Autodesk Inventor part; units mm, degrees
ref_plane "YZ Plane" through (0, 0, 0) normal (1, 0, 0) x (0, 1, 0)
ref_plane "XZ Plane" through (0, 0, 0) normal (0, 1, 0) x (-1, 0, 0)
ref_plane "XY Plane" through (0, 0, 0) normal (0, 0, 1) x (1, 0, 0)
sketch "Sketch1" plane through (0, 0, 0) normal (1, 0, 0) x (0, 1, 0)
  circle A0 centre (0, 0) radius 1.5
  line L0 (0, 0) -> (-35.6, 0)
  circle A1 centre (-35.6, 0) radius 1.5
  line L1 (0, 0) -> (0, -51.5)
  circle A2 centre (0, -51.5) radius 1.5
  circle A3 centre (-35.6, -51.5) radius 1.5
  line L2 (0, 0) -> (-35.6, 0)
  line L3 (-35.6, 0) -> (-35.6, -51.5)
  line L4 (-35.6, -51.5) -> (0, -51.5)
  line L5 (0, -51.5) -> (0, 0)
  line L6 (-17.8, 0) -> (-17.8, -51.5)
  line L7 (-17.8, -25.75) -> (-17.8, 0)
  line L8 (-17.8, -12.875) -> (-17.8, -51.5)
  line L9 (-17.8, -25.75) -> (-17.8, -51.5)
  line L10 (-17.8, -38.625) -> (-17.8, -12.875)
  circle A4 centre (-17.8, -12.875) radius 2.25
  circle A5 centre (-17.8, -38.625) radius 2.25
  line L11 (-15.9797, -9.3512) -> (-0.86, 1.229)
  line L12 (-19.6203, -9.3512) -> (-34.74, 1.229)
  line L13 (-15.55, -15.4984) -> (-15.55, -36.0016)
  line L14 (-20.05, -36.0016) -> (-20.05, -15.4984)
  line L15 (-19.6203, -42.1488) -> (-34.74, -52.729)
  line L16 (-21.2808, -38.5117) -> (-36.5185, -50.3141)
  line L17 (-21.2808, -12.9883) -> (-36.5185, -1.1859)
  line L18 (-14.3192, -12.9883) -> (0.9185, -1.1859)
  line L19 (-14.3192, -38.5117) -> (0.9185, -50.3141)
  line L20 (-15.9797, -42.1488) -> (-0.86, -52.729)
  arc A6 (-14.3192, -12.9883) -> (-15.55, -15.4984) centre (-12.375, -15.4984) ccw
  arc A7 (-15.55, -36.0016) -> (-14.3192, -38.5117) centre (-12.375, -36.0016) ccw
  arc A8 (-21.2808, -38.5117) -> (-20.05, -36.0016) centre (-23.225, -36.0016) ccw
  arc A9 (-20.05, -15.4984) -> (-21.2808, -12.9883) centre (-23.225, -15.4984) ccw
  arc A10 (-19.6203, -9.3512) -> (-15.9797, -9.3512) centre (-17.8, -6.7499) ccw
  arc A11 (-15.9797, -42.1488) -> (-19.6203, -42.1488) centre (-17.8, -44.7501) ccw
  line L21 (1.6962, -2.1899) -> (-13.5415, -13.9923)
  arc A12 (-13.5415, -13.9923) -> (-14.28, -15.4984) centre (-12.375, -15.4984) ccw
  line L22 (-14.28, -15.4984) -> (-14.28, -36.0016)
  arc A13 (-14.28, -36.0016) -> (-13.5415, -37.5077) centre (-12.375, -36.0016) ccw
  line L23 (-13.5415, -37.5077) -> (1.6962, -49.3101)
  line L24 (-37.2962, -2.1899) -> (-22.0585, -13.9923)
  arc A14 (-21.32, -15.4984) -> (-22.0585, -13.9923) centre (-23.225, -15.4984) ccw
  line L25 (-21.32, -15.4984) -> (-21.32, -36.0016)
  arc A15 (-22.0585, -37.5077) -> (-21.32, -36.0016) centre (-23.225, -36.0016) ccw
  line L26 (-22.0585, -37.5077) -> (-37.2962, -49.3101)
  line L27 (-1.5881, 2.2695) -> (-16.7078, -8.3107)
  arc A16 (-18.8922, -8.3107) -> (-16.7078, -8.3107) centre (-17.8, -6.7499) ccw
  line L28 (-18.8922, -8.3107) -> (-34.0119, 2.2695)
  circle A17 centre (0, 0) radius 2.77
  circle A18 centre (-17.8, -12.875) radius 3.52
  circle A19 centre (-17.8, -38.625) radius 3.52
  circle A20 centre (-35.6, 0) radius 2.77
  circle A21 centre (-35.6, -51.5) radius 2.77
  circle A22 centre (0, -51.5) radius 2.77
  line L29 (-1.5881, -53.7695) -> (-16.7078, -43.1893)
  arc A23 (-16.7078, -43.1893) -> (-18.8922, -43.1893) centre (-17.8, -44.7501) ccw
  line L30 (-18.8922, -43.1893) -> (-34.0119, -53.7695)
  point P0 (-17.8, -10.625)
  point P1 (-15.55, -12.875)
  point P2 (-15.55, -38.625)
  point P3 (-20.05, -38.625)
  point P4 (-20.05, -12.875)
  point P5 (-17.8, -40.875)
  point P6 (-18.8754, -36.6486)
  point P7 (-18.8754, -14.8514)
  point P8 (-16.7246, -14.8514)
  point P9 (-16.7246, -36.6486)
  point P10 (-34.0119, 2.2695)
  point P11 (1.6962, -49.3101)
  dimension "d0" = 3
  dimension "d1" = 35.6
  dimension "d2" = 51.5
  dimension "d3" = 4.5
  dimension "d4" = 3.175
  dimension "d5" = 1.27
  dimension "d6" = 1.27
  dimension "d7" = 1.27
  dimension "d8" = 1.27
  dimension "d9" = 1.27
  dimension "d10" = 1.27
  dimension "d11" = 1.27
  dimension "d12" = 1.27
  dimension "d13" = 1.27
  dimension "d14" = 1.27
extrude "Extrusion1" add sketch "Sketch1" along normal blind 2.54 contours A0 L11 L0 A17 L1 L18 | A0 L0 L11 | L18 L1 A0 | A0 L1 L18 A17 L11 L0 | L11 A17 L0 | L1 A17 L18 | A17 L11 A10 A18 L6 A16 L27 L0 | L0 L27 A17 | A17 L18 A18 A10 L11 | A17 L21 L1 | L1 L21 A12 L22 A13 L23 A22 L19 A19 L13 A18 L18 A17 | A18 L13 A6 L18 | L18 A6 L13 A18 L6 A4 A10 | A10 L6 A18 | L23 A22 L1 | L13 A19 L6 A18 | L28 A16 L6 A18 A10 L12 A20 L0 | L0 A20 L28 | A10 A18 L6 | L6 A4 A18 L14 A9 L17 A10 | A22 L4 L20 A2 L19 L1 | L1 L19 A22 | A19 L19 A7 L13 | L13 A7 L19 A19 A11 L6 A5 | L6 A19 L14 A18 | A20 L12 L0 | L0 L12 A1 L17 L3 A20 | A18 L17 A20 L12 A10 | L19 A2 L1 | L1 A2 L4 L20 A22 L19 | A22 L20 A11 A19 L19 | L6 A5 A11 A19 L16 A8 L14 | A18 L17 A9 L14 | L14 A19 L16 A21 L3 L26 A15 L25 A14 L24 A20 L17 A18 | L12 A20 L17 L3 A1 L0 | L0 A1 L12 | A20 L3 L24 | A22 L4 L29 A23 L6 A19 A11 L20 | L20 L4 A22 | L29 L4 A22 | L14 A8 L16 A19 | A20 L3 L17 | A2 L20 L4 | A19 L6 A11 | A19 A11 L15 A21 L16 | L3 L17 A1 | L3 A21 L26 | L6 A19 A11 | L6 A23 L30 L4 A21 L15 A11 A19 | A21 L15 L4 A3 L3 L16 | L16 L3 A21 | L3 L16 A3 L15 L4 A21 | L30 A21 L4 | L3 A3 L16 | A21 L4 L15 | L15 A3 L4
sketch "Sketch2" plane through (2.54, 0, 0) normal (1, 0, 0) x (0, 0, -1)
  circle A0 centre (0, 0) radius 1.5
  circle A1 centre (0, 0) radius 1.5
  circle A2 centre (12.875, -17.8) radius 2.25
  circle A3 centre (12.875, -17.8) radius 2.25
  circle A4 centre (38.625, -17.8) radius 2.25
  circle A5 centre (38.625, -17.8) radius 2.25
  circle A6 centre (51.5, 0) radius 1.5
  circle A7 centre (51.5, 0) radius 1.5
  circle A8 centre (51.5, -35.6) radius 1.5
  circle A9 centre (51.5, -35.6) radius 1.5
  circle A10 centre (0, -35.6) radius 1.5
  circle A11 centre (0, -35.6) radius 1.5
  line L0 (13.9923, -13.5415) -> (2.1899, 1.6962)
  arc A12 (2.1899, 1.6962) -> (-2.2695, -1.5881) centre (0, 0) ccw
  arc A13 (2.1899, 1.6962) -> (-2.2695, -1.5881) centre (0, 0) ccw
  arc A14 (53.7695, -1.5881) -> (49.3101, 1.6962) centre (51.5, 0) ccw
  arc A15 (53.7695, -1.5881) -> (49.3101, 1.6962) centre (51.5, 0) ccw
  arc A16 (49.3101, -37.2962) -> (53.7695, -34.0119) centre (51.5, -35.6) ccw
  arc A17 (49.3101, -37.2962) -> (53.7695, -34.0119) centre (51.5, -35.6) ccw
  arc A18 (-2.2695, -34.0119) -> (2.1899, -37.2962) centre (0, -35.6) ccw
  arc A19 (-2.2695, -34.0119) -> (2.1899, -37.2962) centre (0, -35.6) ccw
  arc A20 (15.4984, -21.32) -> (13.9923, -22.0585) centre (15.4984, -23.225) ccw
  arc A21 (15.4984, -21.32) -> (13.9923, -22.0585) centre (15.4984, -23.225) ccw
  arc A22 (8.3107, -18.8922) -> (8.3107, -16.7078) centre (6.7499, -17.8) ccw
  arc A23 (8.3107, -18.8922) -> (8.3107, -16.7078) centre (6.7499, -17.8) ccw
  arc A24 (13.9923, -13.5415) -> (15.4984, -14.28) centre (15.4984, -12.375) ccw
  arc A25 (13.9923, -13.5415) -> (15.4984, -14.28) centre (15.4984, -12.375) ccw
  arc A26 (36.0016, -14.28) -> (37.5077, -13.5415) centre (36.0016, -12.375) ccw
  arc A27 (36.0016, -14.28) -> (37.5077, -13.5415) centre (36.0016, -12.375) ccw
  arc A28 (37.5077, -22.0585) -> (36.0016, -21.32) centre (36.0016, -23.225) ccw
  arc A29 (37.5077, -22.0585) -> (36.0016, -21.32) centre (36.0016, -23.225) ccw
  arc A30 (43.1893, -16.7078) -> (43.1893, -18.8922) centre (44.7501, -17.8) ccw
  arc A31 (43.1893, -16.7078) -> (43.1893, -18.8922) centre (44.7501, -17.8) ccw
  line L1 (2.1899, 1.6962) -> (13.9923, -13.5415)
  line L2 (-2.2695, -1.5881) -> (8.3107, -16.7078)
  line L3 (8.3107, -16.7078) -> (-2.2695, -1.5881)
  line L4 (8.3107, -18.8922) -> (-2.2695, -34.0119)
  line L5 (8.3107, -18.8922) -> (-2.2695, -34.0119)
  line L6 (2.1899, -37.2962) -> (13.9923, -22.0585)
  line L7 (15.4984, -21.32) -> (36.0016, -21.32)
  line L8 (36.0016, -14.28) -> (15.4984, -14.28)
  line L9 (36.0016, -14.28) -> (15.4984, -14.28)
  line L10 (49.3101, 1.6962) -> (37.5077, -13.5415)
  line L11 (49.3101, 1.6962) -> (37.5077, -13.5415)
  line L12 (43.1893, -16.7078) -> (53.7695, -1.5881)
  line L13 (53.7695, -34.0119) -> (43.1893, -18.8922)
  line L14 (43.1893, -18.8922) -> (53.7695, -34.0119)
  line L15 (37.5077, -22.0585) -> (49.3101, -37.2962)
  arc A32 (-4.3506, -32.5556) -> (4.198, -38.8516) centre (0, -35.6) ccw
  line L16 (-4.3506, -32.5556) -> (5.9748, -17.8)
  line L17 (5.9748, -17.8) -> (-4.3506, -3.0444)
  arc A33 (4.198, 3.2516) -> (-4.3506, -3.0444) centre (0, 0) ccw
  line L18 (4.198, 3.2516) -> (15.8097, -11.74)
  line L19 (15.8097, -11.74) -> (35.6903, -11.74)
  line L20 (35.6903, -11.74) -> (47.302, 3.2516)
  arc A34 (55.8506, -3.0444) -> (47.302, 3.2516) centre (51.5, 0) ccw
  line L21 (47.302, -38.8516) -> (35.6903, -23.86)
  line L22 (35.6903, -23.86) -> (15.8097, -23.86)
  line L23 (15.8097, -23.86) -> (4.198, -38.8516)
  arc A35 (-4.3506, -32.5556) -> (4.198, -38.8516) centre (0, -35.6) ccw
  line L24 (35.4996, -11.9862) -> (47.302, 3.2516)
  arc A36 (55.8506, -3.0444) -> (47.302, 3.2516) centre (51.5, 0) ccw
  line L25 (55.8506, -3.0444) -> (45.5252, -17.8)
  line L26 (45.5252, -17.8) -> (55.8506, -32.5556)
  circle A37 centre (51.5, -35.6) radius 5.31
  point P0 (55.8506, -3.0444)
  point P1 (4.198, -38.8516)
  dimension "d17" = 2.54
  dimension "d18" = 2.54
  dimension "d19" = 2.54
extrude "Extrusion2" add sketch "Sketch2" against normal up to surface (2.54 mm away)
fillet "Fillet1" radius 12.7 6 edges at (1.27, -17.8, -5.9748) (1.27, -23.86, -15.8097) (1.27, -23.86, -35.6903) (1.27, -17.8, -45.5252) (1.27, -11.74, -35.6903) (1.27, -11.74, -15.8097)
properties part number "pump mount_3DPrint"
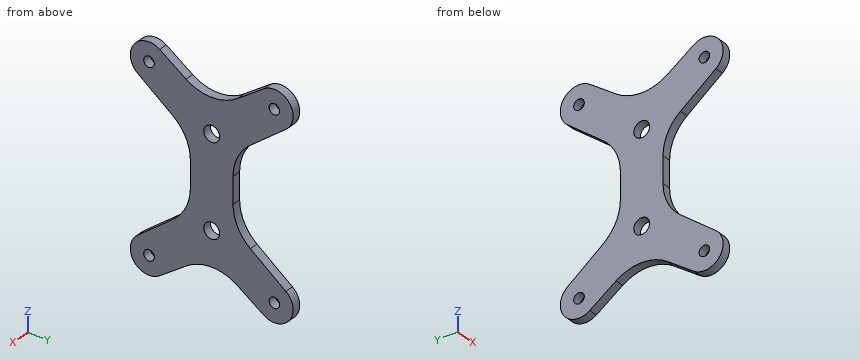
Geometry check sheet. Reference: the model listing, model coordinates, mm. Coordinates: 2 decimals unless noted, no trailing zeros. Write each loop counter-clockwise with the first axis right and the second up, starting at its lowest first coordinate (ties: lowest second). Pieces come first, ordered by that corner, then holes. Notation, with made-up numbers: (-2.75, 75) -> (18.25, 75) arc R18 cw to (18.25, 84) -> close; hole circle Ø4 at (89, 19). An arc over 180 degrees is marked (long way). One line per question, with ' | ' between items.
1. Thickness scan on probe 1 along Y at (x, z) = (1.15, 0); probe 2 along Z at (x, y) = (2, -35.6); probe 3 along Z at (x, y) = (1.75, 0.5). Record the ranges inside material, lowest first. Write a range as from..to.
Answers:
probe 1: y = -40.91..-37.1, -34.1..-26.34, -9.26..-1.5, 1.5..5.31 | probe 2: z = -56.81..-53, -50..-44.78, -6.72..-1.5, 1.5..5.31 | probe 3: z = -56.79..-52.91, -50.09..-45.17, -6.33..-1.41, 1.41..5.29
2. Depth check by flat-ended pin: pin 1 Ø1 at (x, y) = (2, -31) entering from -Z; pin 2 Ø1 at (x, z) = (2, -12) entering from -Y; pin 3 Ø3.5 at (y, z) = (-17.8, -12.875) entering from +X. Enter the tip coordinate at first touch or a pass-through.
Answers:
pin 1: stops at z = -55.11 | pin 2: stops at y = -29.42 | pin 3: passes through
3. Cross-section at C-C on z = 0. Record the cut outline in (x, y).
Answers:
outline: (0, -40.91) -> (2.54, -40.91) -> (2.54, -37.1) -> (0, -37.1) -> close; (0, -34.1) -> (2.54, -34.1) -> (2.54, -26.34) -> (0, -26.34) -> close; (0, -9.26) -> (2.54, -9.26) -> (2.54, -1.5) -> (0, -1.5) -> close; (0, 1.5) -> (2.54, 1.5) -> (2.54, 5.31) -> (0, 5.31) -> close
4. Cross-section at D-D on x = 0.9. Record the cut outline in (y, z) (3 decimals).
Answers:
outline: (-38.852, -47.302) arc R5.31 ccw to (-32.556, -55.851) -> (-25.081, -50.62) arc R12.7 cw to (-10.519, -50.62) -> (-3.044, -55.851) arc R5.31 ccw to (3.252, -47.302) -> (-6.817, -39.504) arc R12.7 cw to (-11.74, -29.463) -> (-11.74, -22.037) arc R12.7 cw to (-6.817, -11.996) -> (3.252, -4.198) arc R5.31 ccw to (-3.044, 4.351) -> (-10.519, -0.88) arc R12.7 cw to (-25.081, -0.88) -> (-32.556, 4.351) arc R5.31 ccw to (-38.852, -4.198) -> (-28.783, -11.996) arc R12.7 cw to (-23.86, -22.037) -> (-23.86, -29.463) arc R12.7 cw to (-28.783, -39.504) -> close; hole circle Ø3 at (-35.6, -51.5); hole circle Ø3 at (-35.6, 0); hole circle Ø4.5 at (-17.8, -38.625); hole circle Ø4.5 at (-17.8, -12.875); hole circle Ø3 at (0, -51.5); hole circle Ø3 at (0, 0)
5. Cross-section at A-A on y = -17.8. Record the cut outline in (x, z) (3 decimals).
Answers:
outline: (0, -48.326) -> (2.54, -48.326) -> (2.54, -40.875) -> (0, -40.875) -> close; (0, -36.375) -> (2.54, -36.375) -> (2.54, -15.125) -> (0, -15.125) -> close; (0, -10.625) -> (2.54, -10.625) -> (2.54, -3.174) -> (0, -3.174) -> close
6. Cross-section at B-B on y = -38. Record the cut outline in (x, z), and give its area (3 significant figures).
Answers:
outline: (0, -56.24) -> (2.54, -56.24) -> (2.54, -46.64) -> (0, -46.64) -> close; (0, -4.86) -> (2.54, -4.86) -> (2.54, 4.74) -> (0, 4.74) -> close | area: 48.7 mm²
